Could you check a few things on this model? Use its own coordinates, in mm. A direction names the side the tool comes from. Give positions to 0.01 mm unless a question says otherwise; leave off trailing zeros. Order: outer loops, then holes, each group sorted by start corner. A loop starts at its lowest first (then second) coordinate and runs counter-clockwise, first axis right, second up. Notation, with made-up numbers: (61.5, 48) -> (117.5, 48) arc R14 ccw to (117.5, 57) -> close; hole circle Ø10 at (21.5, -38.75). An arc over 180 degrees is marked (long way). Answer as CSV lines item,"result". Start each with the question number.
(1) I want a section at B-B (x = -20.35). Please give me the cut outline in (y, z), plus the area to 3 significant figures.
(2) Will these pins go through, and if not, where does the flat tip stop? pin 1 Ø1.5 at (y, z) = (3.5, -8.5) entering from -X; pin 2 Ø1 at (x, z) = (-22.5, 3) entering from +Y; pin 3 Ø1.5 at (y, z) = (2, -9) entering from +X.
(3) I need wall thicknesses on L1, parallel to X at y = 11.75, z = 2.75; L2, parallel to Z at x = -15.35, y = 2.9; L3, parallel to Z at x = -20.35, y = 1. Which ranges of each line are inside material? Lowest first, please.
(4) On a 3-axis mill with a long thin cutter (end or side, diameter ignored), from which of +Z, -Z, +X, -X, +Y, -Y can I reach the whole of each face in a straight line? I mean faces 1 (the face through (0, 5, -1)), 2 (the face through (-28, 8, -6)), 3 (the face through (-28, 17, 0)), 4 (the face through (15.3, 3, -9)). Say none if no direction works.
(5) We'd pull the mould along X, two halves only. Please class faces 5 (the face through (25.3, 3, -9)), 6 (the face through (20, 3, -12)), 7 (the face through (19.318, 2.535, -9.653)): released by +X, released by -X, zero draft, split by the parting line, or undercut.
(6) I want a section at A-A (y = 12). Please give me the cut outline in (x, z), plus the area to 3 significant figures.
(7) I want a section at C-C (z = 4.5). Please give me the cut outline in (x, y).
(8) I want a section at D-D (x = 6). Please give me the cut outline in (y, z), plus the area to 3 significant figures.
```python
from build123d import *

# Parameters (mm, degrees)
SKETCH_1_W      = 60
SKETCH_1_H      = 12
EXTRUDE_1_DEPTH = 5
SKETCH_2_W      = 4.7
SKETCH_2_H      = 12
EXTRUDE_2_DEPTH = 12
M3X0_5_3_D      = 2.8
SKETCH_12_W     = 10
SKETCH_12_H     = 6
EXTRUDE_3_DEPTH = 5
M3X0_5_4_D      = 2.8


with BuildPart() as part:
    # 草图1 → 凸台-拉伸1 (new body)
    with BuildSketch(Plane(origin=(0, 0, 0), x_dir=(1, 0, 0), z_dir=(0, 1, 0))):
        Rectangle(SKETCH_1_W, SKETCH_1_H)
    extrude(amount=EXTRUDE_1_DEPTH)

    # 草图2 → 凸台-拉伸2 (add)
    with BuildSketch(Plane(origin=(0, 5, 0), x_dir=(1, 0, 0), z_dir=(0, 1, 0))):
        with Locations((-27.65, 0)):
            Rectangle(SKETCH_2_W, SKETCH_2_H)
        with Locations((27.65, 0)):
            Rectangle(SKETCH_2_W, SKETCH_2_H)
    extrude(amount=EXTRUDE_2_DEPTH)

    # M3x0.5 螺纹孔3 (through all)
    with Locations(Plane(origin=(0, 0, 0), x_dir=(-1, 0, 0), z_dir=(0, -1, 0))):
        with Locations((-15.35, 0), (15.35, 0)):
            Hole(M3X0_5_3_D / 2)

    # 草图12 → 凸台-拉伸3 (add)
    with BuildSketch(Plane(origin=(0, 5, 0), x_dir=(1, 0, 0), z_dir=(0, 1, 0))):
        with Locations((-20.3, 9)):
            Rectangle(SKETCH_12_W, SKETCH_12_H)
        with Locations((20.3, 9)):
            Rectangle(SKETCH_12_W, SKETCH_12_H)
    extrude(amount=-EXTRUDE_3_DEPTH)

    # M3x0.5 螺纹孔4 (through all)
    with Locations(Plane(origin=(0, 0, 0), x_dir=(-1, 0, 0), z_dir=(0, -1, 0))):
        with Locations((20.35, 8.706622657), (-20.35, 8.706622657)):
            Hole(M3X0_5_4_D / 2)


solid = part.part
```
Final values:
1,outline,"(0, -12) -> (5, -12) -> (5, -10.11) -> (0, -10.11) -> close; (0, -7.31) -> (5, -7.31) -> (5, 6) -> (0, 6) -> close"
1,area,"76.0 mm²"
2,pin 1,"x = -25.3"
2,pin 2,"y = 5"
2,pin 3,"x = 25.3"
3,L1,"-30 to -25.3, 25.3 to 30"
3,L2,"-12 to -1.4, 1.4 to 6"
3,L3,"-12 to -10.11, -7.31 to 6"
4,face 1,"+Z, -Z, +Y"
4,face 2,"-Z, -X, +Y, -Y"
4,face 3,"+Z, -Z, +X, -X, +Y"
4,face 4,"-Z, +Y, -Y"
5,face 5,"released by +X"
5,face 6,"zero draft"
5,face 7,"undercut"
6,outline,"(-30, -6) -> (-25.3, -6) -> (-25.3, 6) -> (-30, 6) -> close; (25.3, -6) -> (30, -6) -> (30, 6) -> (25.3, 6) -> close"
6,area,"113 mm²"
7,outline,"(-30, 0) -> (30, 0) -> (30, 17) -> (25.3, 17) -> (25.3, 5) -> (-25.3, 5) -> (-25.3, 17) -> (-30, 17) -> close"
8,outline,"(0, -6) -> (5, -6) -> (5, 6) -> (0, 6) -> close"
8,area,"60.0 mm²"
